Verification items for the finished model (mm, model axes). Face numbers are marked on the shaded views. A direction names the side the tool comes from. Round coordinates to 2 decimals unless told otherwise and drop trailing zeros. Write each loop counter-clockwise with the first axis right and the second up, starting at its lowest first coordinate (ties: lowest second). Pieces come first, ordered by that corner, then holes. Notation, with made-up numbers: M -38.5,15 L -12.5,15 A25 ccw -12.5,54 Z; hole C 87.25,55.5 d2. An arc over 180 degrees is marked long. Use a Markdown table: item, result. Add a question column.
from build123d import *

# Parameters (mm, degrees)
SKETCH3_R           = 10
BOSS_EXTRUDE2_DEPTH = 15
SKETCH4_W           = 20
SKETCH4_H           = 25
CUT_EXTRUDE2_DEPTH  = 15


with BuildPart() as part:
    # Sketch3 → Boss-Extrude2 (new body, symmetric)
    with BuildSketch(Plane.XY):
        with BuildLine():
            Line((0, 12.5), (100, 12.5))
            ThreePointArc((100, 12.5), (112.5, 0), (100, -12.5))
            Line((100, -12.5), (0, -12.5))
            ThreePointArc((0, -12.5), (-12.5, 0), (0, 12.5))
        make_face()
        Circle(SKETCH3_R, mode=Mode.SUBTRACT)
        with Locations((100, 0)):
            Circle(SKETCH3_R, mode=Mode.SUBTRACT)
    extrude(amount=BOSS_EXTRUDE2_DEPTH, both=True)

    # Sketch4 → Cut-Extrude2 (cut, symmetric)
    with BuildSketch(Plane(origin=(0, 0, 0), x_dir=(0, 0, -1), z_dir=(1, 0, 0))):
        Rectangle(SKETCH4_W, SKETCH4_H)
    extrude(amount=CUT_EXTRUDE2_DEPTH, both=True, mode=Mode.SUBTRACT)


solid = part.part
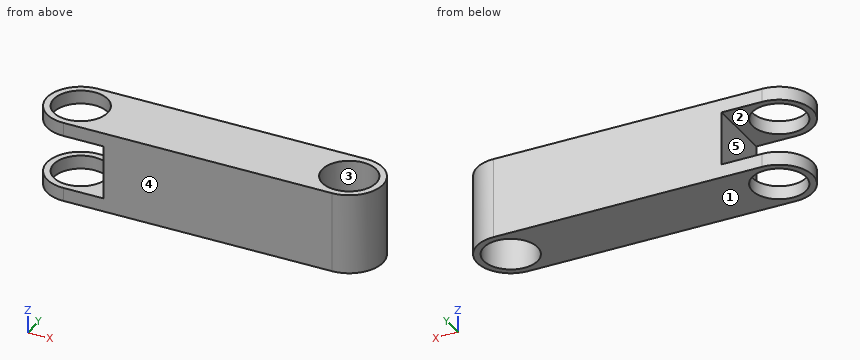
1. Release check for a two-part mould opening along Z. For the marked faces 1, 2 and 3 record: +Z half, -Z half, draft (parallel to the pull), parting line (faces both ways), or undercut.
2. Access from +Z, -Z, +X, -X, +Y, -Y to the whole of each face (thin tool, end or side, straight path). Record for the marked faces 4 and 5.
3. Cross-section at B-B on x = 105.5. Enter the section's corners in (y, z), plus the area to 3 significant figures.
4. Cross-section at D-D on z = -7. Enter the section's corners in (x, y).
5. Depth check by flat-ended pin: pin 1 Ø1.5 at (y, z) = (-4, -11.5) entering from -X; pin 2 Ø10 at (y, z) = (4.5, 3) entering from -X; pin 3 Ø7.5 at (x, y) = (4.5, 1.5) entering from -Z. Enter the tip coordinate at first touch or a pass-through.
6. Cross-section at A-A on y = 0. Enter the section's corners in (x, z).
7. Scan lines: line 1 along Y through (x, z) = (0, 13.75); line 2 along X through (y, z) = (-0.5, -3); line 3 along Z through (x, y) = (11.5, -3.75). Record each from-to range of solid material in increasing order. Write a range as from..to.
8. Cross-section at C-C on z = 12.5. Enter the section's corners in (x, y), plus the area to 3 significant figures.
Answer:
| question | item | result |
|---|---|---|
| 1 | face 1 | -Z half |
| 1 | face 2 | undercut |
| 1 | face 3 | draft |
| 2 | face 4 | +Z, -Z, +X, -X, -Y |
| 2 | face 5 | -X, +Y, -Y |
| 3 | outline | M -11.22,-15 L -8.35,-15 L -8.35,15 L -11.22,15 Z; M 8.35,-15 L 11.22,-15 L 11.22,15 L 8.35,15 Z |
| 3 | area | 172 mm^2 |
| 4 | outline | M 15,-12.5 L 100,-12.5 A12.5 ccw 100,12.5 L 15,12.5 Z; hole C 100,0 d20 |
| 5 | pin 1 | stops at x = -12.07 |
| 5 | pin 2 | stops at x = 15 |
| 5 | pin 3 | passes through |
| 6 | outline | M -12.5,-15 L -10,-15 L -10,-10 L -12.5,-10 Z; M -12.5,10 L -10,10 L -10,15 L -12.5,15 Z; M 10,-15 L 90,-15 L 90,15 L 10,15 L 10,10 L 15,10 L 15,-10 L 10,-10 Z; M 110,-15 L 112.5,-15 L 112.5,15 L 110,15 Z |
| 7 | line 1 | y = -12.5..-10, 10..12.5 |
| 7 | line 2 | x = 15..90.01, 109.99..112.49 |
| 7 | line 3 | z = -15..-10, 10..15 |
| 8 | outline | M 0,-12.5 L 100,-12.5 A12.5 ccw 100,12.5 L 0,12.5 A12.5 ccw Z; hole C 0,0 d20; hole C 100,0 d20 |
| 8 | area | 2,360 mm^2 |
